Autodesk Fusion 360 part; units mm, degrees
sketch "Sketch1" plane through (0, 0, 0) normal (0, 0, 1) x (1, 0, 0)
  line L0 (36, 27) -> (-36, 27)
  line L1 (-36, 27) -> (-36, -27)
  line L2 (-36, -27) -> (36, -27)
  line L3 (36, -27) -> (36, 27)
  line L4 (36, 30.6) -> (-36, 30.6)
  line L5 (-36, 35.6) -> (-36, -30.6)
  line L6 (-36, -30.6) -> (36, -30.6)
  line L7 (36, -30.6) -> (36, 30.6)
  line L8 (33, 35.6) -> (-36, 35.6)
  line L9 (41, -27.6) -> (41, 27.6)
  line L10 (33, -35.6) -> (-36, -35.6)
  line L11 (-36, -35.6) -> (-36, 30.6)
  arc A0 (41, 27.6) -> (33, 35.6) centre (33, 27.6) ccw
  arc A1 (33, -35.6) -> (41, -27.6) centre (33, -27.6) ccw
  circle A2 centre (-20, 0) radius 1.75
  circle A3 centre (15, 0) radius 1.75
  line L12 (-20, 9.5) -> (15, 9.5)
  arc A4 (15, 9.5) -> (15, 17.5) centre (15, 13.5) ccw
  line L13 (15, 17.5) -> (-20, 17.5)
  arc A5 (-20, 17.5) -> (-20, 9.5) centre (-20, 13.5) ccw
  line L14 (-20, 13.5) -> (15, 13.5) construction
  line L15 (1.75, 0) -> (22.5, 0)
  line L16 (-20, -9.5) -> (15, -9.5)
  line L17 (15, -17.5) -> (-20, -17.5)
  arc A6 (15, -17.5) -> (15, -9.5) centre (15, -13.5) ccw
  arc A7 (-20, -9.5) -> (-20, -17.5) centre (-20, -13.5) ccw
  dimension "d1" = 72
  dimension "d2" = 54
  dimension "d3" = 61.2
  dimension "d6" = 8
  dimension "d32" = 3.5
  dimension "d33" = 3.5
  dimension "d34" = 8
extrude "Extrude1" add sketch "Sketch1" along normal blind 6.4 contours L3 L4 L5 L6 L7 L8 L9 L10 L11 A0 A1 | L0 L4 L5 L7 L11 | L2 L5 L6 L7 L11
extrude "Extrude2" add sketch "Sketch1" along normal blind 24 contours L3 L4 L5 L6 L7 L8 L9 L10 L11 A0 A1
extrude "Extrude3" add sketch "Sketch1" along normal blind 27 and the other way blind -24
sketch "Sketch2" plane through (0, -35.6, 0) normal (0, -1, 0) x (1, 0, 0)
  line L0 (-36, 0) -> (33, 0)
  line L1 (33, 0) -> (33, 27)
  line L2 (-36, 27) -> (-36, 0)
  line L3 (-36, 0) -> (-49.5029, 27)
  line L4 (-36, 0) -> (-6, 0) construction
  line L5 (-36, 27) -> (-49.5029, 27)
  line L6 (33, 27) -> (-36, 27)
  line L7 (-36, 27) -> (-36, 24)
  line L8 (-36, 24) -> (-36.4845, 24)
  line L9 (-36.4845, 24) -> (-48.0026, 24)
  line L10 (-36, 0) -> (-36, 6.4)
  line L11 (-36, 6.4) -> (-36, 6)
  line L12 (-36, 6.4) -> (-39.2007, 6.4)
  dimension "d11" = 116.57
  dimension "d25" = 6.4
extrude "Extrude4" add sketch "Sketch2" against normal blind 5 contours L2 L3 L10 L11 L12 | L2 L3 L8 L9 L12
extrude "Extrude5" add sketch "Sketch2" along normal blind -71.2 and the other way blind 66.2 contours L2 L3 L10 L11 L12 | L2 L3 L8 L9 L12
extrude "Extrude6" add sketch "Sketch2" against normal blind 71.2 contours L2 L3 L5 L7 L8 L9
extrude "Extrude7" add sketch "Sketch2" against normal blind 8.6 contours L2 L3 L10 L11 L12
extrude "Extrude8" add sketch "Sketch2" along normal blind -66.2 and the other way blind 62.6 contours L2 L3 L10 L11 L12
chamfer "Chamfer1" distance 1 angle 45 2 edges at (-21.6316, 0.6328, 24) (13.3684, 0.6328, 24)
Verification items for the finished model (mm, model axes). A direction names the side the tool comes from. Coordinates: 2 decimals unless noted, no trailing zeros. Order: outer loops, then holes, each group sorted by start corner. A loop starts at its lowest first (then second) coordinate and runs counter-clockwise, first axis right, second up. Notation, with made-up numbers: M 82,2.5 L 107,2.5 A24 cw 107,28.5 Z; hole C 45.5,-9 d9. An arc over 180 degrees is marked long. Write each question's results on one line, items separated by ' | '.
1) Section check C-C on z = 22. Record the cut outline in (x, y), plus the area to 3 significant figures.
Solved:
outline: M -47,-35.6 L 33,-35.6 A8 ccw 41,-27.6 L 41,27.6 A8 ccw 33,35.6 L -47,35.6 L -47,30.6 L 36,30.6 L 36,-30.6 L -47,-30.6 Z | area: 1,160 mm²
2) Section check B-B on y = 0. Record the cut outline in (x, z), plus the area to 3 significant figures.
Solved:
outline: M -49.5,27 L -48,24 L -22.75,24 L -21.75,25 L -21.75,27 Z; M -18.25,25 L -17.25,24 L 12.25,24 L 13.25,25 L 13.25,27 L -18.25,27 Z; M 16.75,25 L 17.75,24 L 36,24 L 36,0 L 41,0 L 41,27 L 16.75,27 Z | area: 366 mm²
3) Section check A-A on x = 3. Record the cut outline in (y, z).
Solved:
outline: M -35.6,0 L -27,0 L -27,6.4 L -30.6,6.4 L -30.6,24 L -17.5,24 L -17.5,27 L -35.6,27 Z; M -9.5,24 L 9.5,24 L 9.5,27 L -9.5,27 Z; M 17.5,24 L 30.6,24 L 30.6,6.4 L 27,6.4 L 27,0 L 35.6,0 L 35.6,27 L 17.5,27 Z
4) Release check for a two-part mould opening along X. For faces 1 (the face through (38.719, -33.194, 13.311)), 2 (the face through (-24, 13.4, 25.5)), 3 (the face through (-5, 0, 24)) record: pulls with the +X half, pulls with the -X half, needs draft (parallel to the pull), parting line crosses it, or undercut.
Solved:
face 1: pulls with the +X half | face 2: undercut | face 3: needs draft
5) Section check D-D on y = 13.5. Record the cut outline in (x, z), plus the area to 3 significant figures.
Solved:
outline: M -49.5,27 L -48,24 L -24,24 L -24,27 Z; M 19,24 L 36,24 L 36,0 L 41,0 L 41,27 L 19,27 Z | area: 260 mm²
6) Scan lines: line 1 along Y through (x, z) = (15, 26.15); line 2 along Y through (x, z) = (-16.5, 16); line 3 along Z through (x, y) = (-35.5, -30). Record each from-to range of solid material in increasing order. Write a range as [from, to].
Solved:
line 1: y = [-35.6, -17.5], [-9.5, -1.75], [1.75, 9.5], [17.5, 35.6] | line 2: y = [-35.6, -30.6], [30.6, 35.6] | line 3: z = [0, 6.4], [24, 27]
7) Access from +Z, -Z, +X, -X, +Y, -Y to the whole of each face (thin tool, end or side, straight path). Record for faces 4 (the face through (-2, -27, 3)), 5 (the face through (-7, -30.6, 15)), 6 (the face through (38.594, 33.319, 13.311)), 7 (the face through (19, -13.4, 25.5)), 8 (the face through (-9, 35.6, 14)).
Solved:
face 4: -Z, -X | face 5: -X | face 6: +Z, -Z, +X, +Y | face 7: +Z, -Z | face 8: +Z, -Z, +X, -X, +Y
8) Gauge pin test, flat ends, axial feed: pin 1 Ø3 at (x, y) = (-20, 0) entering from -Z; pin 2 Ø7 at (y, z) = (-4, 14.5) entering from -X. Record the tip position at first contact, or that the pin passes through.
Solved:
pin 1: passes through | pin 2: stops at x = 36
